Print and shaded views of the part. All mm, measured from the part's lowest x, y and z. A direction names the side the tool comes from. Round coordinates to 2 decimals unless told otherwise and drop trailing zeros. Order: outer loops, then holes, each group sorted by start corner. A loop starts at its lowest first (then second) coordinate and runs counter-clockwise, first axis right, second up. Notation, with made-up numbers: M 27,63 L 50,63 A18 cw 50,80 Z; hole C -7,-19 d8. An arc over 180 degrees is marked long. Write each question's results on one line, items separated by ' | '. Start each with the question number.
1. Band-saw the part on D-D, the plane y = 12.5. List the corners of the cut face in (x, z).
2. Band-saw the part on B-B, the plane z = 2.25. List the corners of the cut face in (x, y), then the cut area to 3 significant figures.
3. Which spindle directions (+Z, -Z, +X, -X, +Y, -Y) get a long thin tool onto all of the face, cutting with end or side? Do the marked faces 1 and 2. Say none if no direction does.
4. Two-plate mould, pull along Y, no slides. Class the marked faces 3, 4 and 5: +Y half, -Y half, draft (parallel to the pull), parting line (faces both ways), or undercut.
5. Band-saw the part on C-C, the plane x = 12.5. List the corners of the cut face in (y, z).
6. Drop flat-ended pins along their axis: pin 1 Ø1 at (y, z) = (21.5, 11) entering from +X (1 decimal); pin 2 Ø5 at (x, z) = (22.5, 3) entering from -Y; pin 3 Ø2 at (x, z) = (7, 6.5) entering from +Y. Give the stop position or say it passes through.
7. Probe L1, parallel to X at y = 15.5, z = 9.75 (1 decimal); L2, parallel to X at y = 12.75, z = 2.75; L3, parallel to Y at x = 12.5, z = 13.75 (1 decimal). List the from-to ranges inside material, lowest first. Write a range as [from, to].
8. Band-saw the part on A-A, the plane y = 20.5. List the corners of the cut face in (x, z) (1 decimal), then the cut area to 3 significant figures.
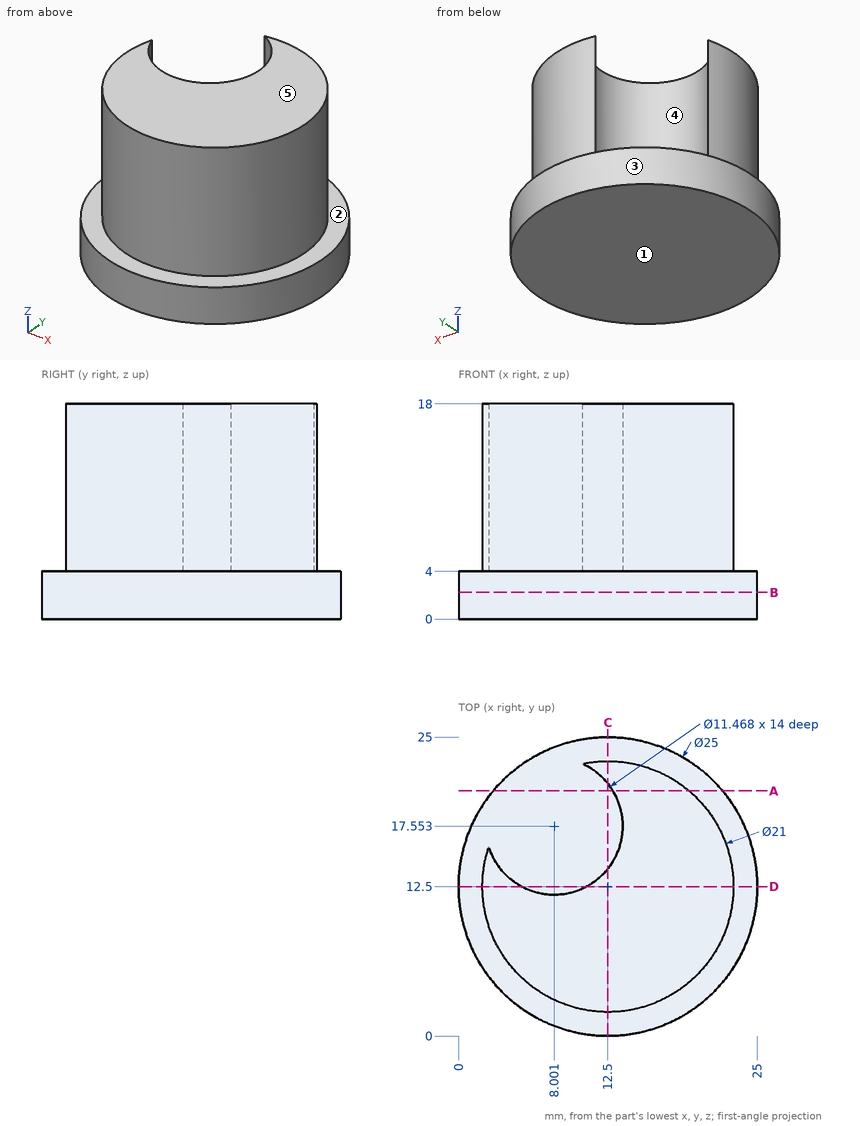
Solution:
1) outline: M 0,0 L 25,0 L 25,4 L 23,4 L 23,18 L 10.71,18 L 10.71,4 L 5.29,4 L 5.29,18 L 2,18 L 2,4 L 0,4 Z
2) outline: C 12.5,12.5 d25 | area: 491 mm^2
3) face 1: -Z, +X, -X, +Y, -Y | face 2: +Z
4) face 3: parting line | face 4: undercut | face 5: draft
5) outline: M 0,0 L 25,0 L 25,4 L 23,4 L 23,18 L 21.11,18 L 21.11,4 L 14,4 L 14,18 L 2,18 L 2,4 L 0,4 Z
6) pin 1: x = 18.7 | pin 2: y = 2.5 | pin 3: y = 12.18
7) L1: [2.4, 2.6], [13.4, 22.6] | L2: [0, 25] | L3: [2, 14], [21.1, 23]
8) outline: M 2.9,0 L 22.1,0 L 22.1,4 L 19.3,4 L 19.3,18 L 12.9,18 L 12.9,4 L 2.9,4 Z | area: 166 mm^2
